from build123d import *

# Parameters (mm, degrees)
SKETCH1_W           = 342
SKETCH1_H           = 657
BOSS_EXTRUDE1_DEPTH = 12
SKETCH2_W           = 6
SKETCH2_H           = 6
CUT_EXTRUDE1_DEPTH  = 475.362993919
CHAMFER1_SIZE       = 6
SKETCH3_R           = 2.6
CUT_EXTRUDE2_DEPTH  = 371.536435455
CHAMFER2_SIZE       = 2.9
SKETCH4_R           = 6
CUT_EXTRUDE3_DEPTH  = 6
SKETCH5_W           = 342
SKETCH5_H           = 48
CUT_EXTRUDE4_DEPTH  = 2


with BuildPart() as part:
    # Sketch1 → Boss-Extrude1 (new body)
    with BuildSketch(Plane.XY):
        Rectangle(SKETCH1_W, SKETCH1_H)
    extrude(amount=BOSS_EXTRUDE1_DEPTH)

    # Sketch2 → Cut-Extrude1 (cut, through all)
    with BuildSketch(Plane.ZY.offset(171)):
        with Locations((9, 325.5)):
            Rectangle(SKETCH2_W, SKETCH2_H)
    extrude(amount=-CUT_EXTRUDE1_DEPTH, mode=Mode.SUBTRACT)

    # Chamfer1
    chamfer1_edges = [part.edges().sort_by_distance(p)[0] for p in [
        (171, 0, 0),
        (-171, 0, 0),
    ]]
    chamfer(chamfer1_edges, length=CHAMFER1_SIZE - 0.0001)  # a hair under: the kernel refuses the full size

    # Sketch3 → Cut-Extrude2 (cut, through all)
    with BuildSketch(Plane(origin=(0, 0, 0), x_dir=(-1, 0, 0), z_dir=(0, 0, -1))):
        with Locations((-71, -303.5)):
            Circle(SKETCH3_R)
        with Locations((71, -303.5)):
            Circle(SKETCH3_R)
        with Locations((71, 296.5)):
            Circle(SKETCH3_R)
        with Locations((-71, 296.5)):
            Circle(SKETCH3_R)
    extrude(amount=-CUT_EXTRUDE2_DEPTH, mode=Mode.SUBTRACT)

    # Chamfer2
    chamfer2_edges = [part.edges().sort_by_distance(p)[0] for p in [
        (73.6, -303.5, 12),
        (-68.4, -303.5, 12),
        (-68.4, 296.5, 12),
        (73.6, 296.5, 12),
    ]]
    chamfer(chamfer2_edges, length=CHAMFER2_SIZE)

    # Sketch4 → Cut-Extrude3 (cut)
    with BuildSketch(Plane(origin=(0, 0, 0), x_dir=(-1, 0, 0), z_dir=(0, 0, -1))):
        with Locations((-91, 296.5)):
            Circle(SKETCH4_R)
        with Locations((-51, 296.5)):
            Circle(SKETCH4_R)
        with Locations((51, 296.5)):
            Circle(SKETCH4_R)
        with Locations((91, 296.5)):
            Circle(SKETCH4_R)
    extrude(amount=-CUT_EXTRUDE3_DEPTH, mode=Mode.SUBTRACT)

    # Sketch5 → Cut-Extrude4 (cut)
    with BuildSketch(Plane(origin=(0, 0, 0), x_dir=(-1, 0, 0), z_dir=(0, 0, -1))):
        with Locations((0, 304.5)):
            Rectangle(SKETCH5_W, SKETCH5_H)
    extrude(amount=-CUT_EXTRUDE4_DEPTH, mode=Mode.SUBTRACT)


solid = part.part
Source: CAD feature listing. Evaluate the final solid. Frame: model axes, mm. A direction names the side the tool comes from. Coordinates: 2 decimals unless noted, no trailing zeros. Order: outer loops, then holes, each group sorted by start corner. A loop starts at its lowest first (then second) coordinate and runs counter-clockwise, first axis right, second up.
Item 1: Cut plane A-A (x = -91). Return loops of the section in (y, z), plus the area to 3 significant figures.
Output values:
outline: (-328.5, 0) - (280.5, 0) - (280.5, 2) - (290.5, 2) - (290.5, 6) - (302.5, 6) - (302.5, 2) - (328.5, 2) - (328.5, 6) - (322.5, 6) - (322.5, 12) - (-328.5, 12) - close
area: 7,700 mm2
Item 2: Material intervals for line 1 (Y direction, x = -71, z = 7.5); line 2 (Y direction, x = 71, z = 4.25); line 3 (X direction, y = 296.5, z = 7), sorted ascending.
Output values:
line 1: y = -328.5 to -306.1, -300.9 to 293.9, 299.1 to 322.5
line 2: y = -328.5 to -306.1, -300.9 to 293.9, 299.1 to 328.5
line 3: x = -171 to -73.6, -68.4 to 68.4, 73.6 to 171
Item 3: Set-up query: faces 4 (the face through (51.78, 302.45, 3.97)), 5 (the face through (2, 305, 2)), 6 (the face through (-2, -328.5, 6)). Return all of +Z, -Z, +X, -X, +Y, -Y with unobstructed straight access to the full face (end or side cutting, diameter ignored); none if empty.
Output values:
face 4: -Z
face 5: -Z, +X, -X, +Y
face 6: +Z, -Z, +X, -X, -Y
Item 4: Cut plane B-B (x = 127). Return loops of the section in (y, z), plus the area to 3 significant figures.
Output values:
outline: (-328.5, 0) - (280.5, 0) - (280.5, 2) - (328.5, 2) - (328.5, 6) - (322.5, 6) - (322.5, 12) - (-328.5, 12) - close
area: 7,750 mm2
Item 5: First-contact query: P1, Ø7, axis at x = -51, y = 296.5, coming from the -Z side; P2, Ø1.6, axis at x = 54.5, z = 0.5, coming from the +Y side; P3, Ø13, axis at x = 52.5, y = 298, coming from the -Z side; P4, Ø6, axis at x = 71, y = -303.5, coming from the -Z side. Flat tips, straight axial feed; report the tip coordinate or a pass-through.
Output values:
P1: stops at z = 6
P2: stops at y = 280.5
P3: stops at z = 2
P4: stops at z = 0
Item 6: Pull-direction query (X, two-part tool) for faces 1 (the face through (-90.22, 302.45, 3.97)), 2 (the face through (-2, -20, 0)), 3 (the face through (51, 297, 6)); classes: pulls with the +X half, pulls with the -X half, needs draft (parallel to the pull), parting line crosses it, or undercut.
Output values:
face 1: undercut
face 2: needs draft
face 3: undercut
